Check sheet for the modelled part. Datum: model origin and axes. Units: mm. Face numbers are marked on the shaded views. A direction names the side the tool comes from. Coordinates: 2 decimals unless noted, no trailing zeros. Order: outer loops, then holes, each group sorted by start corner. A loop starts at its lowest first (then second) coordinate and runs counter-clockwise, first axis right, second up.
1. Draft check along X on the marked faces 3, 4, 5 and 6. Enter one of: released by +X, released by -X, zero draft, split by the parting line, or undercut.
2. Cross-section at A-A (y = 0). Enter the section's corners in (x, z), then the cut area to 3 significant figures.
3. Cross-section at B-B (x = -4.4). Enter the section's corners in (y, z), then the cut area to 3 significant figures.
4. Cross-section at C-C (y = -7.7). Enter the section's corners in (x, z), then the cut area to 3 significant figures.
5. Set-up check for the marked faces 1 and 2: record each of +Z, -Z, +X, -X, +Y, -Y from which the full face is reachable in a straight line by a thin tool's end or side.
6. Thickness scan on line 1 (Y direction, x = 0, z = 0.7); line 2 (X direction, y = 4.5, z = 5); line 3 (Y direction, x = -4.4, z = 0.9). Record the ranges inside material, lowest first.
7. Gauge pin test, flat ends, axial feed: pin 1 Ø1.6 at (x, y) = (-6.22, 0) entering from -Z; pin 2 Ø2.5 at (x, y) = (0, 6.22) entering from +Z; pin 3 Ø3 at (x, y) = (2.5, -1.5) entering from -Z. Record the tip position at first contact, or that the pin passes through.
8. Cross-section at D-D (z = 3.5). Enter the section's corners in (x, y).
Autodesk Inventor part; units mm, degrees
ref_plane "YZ Plane" through (0, 0, 0) normal (1, 0, 0) x (0, 1, 0)
ref_plane "XZ Plane" through (0, 0, 0) normal (0, 1, 0) x (-1, 0, 0)
ref_plane "XY Plane" through (0, 0, 0) normal (0, 0, 1) x (1, 0, 0)
sketch "スケッチ1" plane through (0, 0, 0) normal (0, 0, 1) x (1, 0, 0)
  line L0 (11, -10) -> (-11, -10)
  line L1 (-11, -10) -> (-11, 10)
  line L2 (-11, 10) -> (11, 10)
  line L3 (11, 10) -> (11, -10)
  line L4 (11, -10) -> (-11, 10) construction
  line L5 (-11, -10) -> (11, 10) construction
  point P0 (0, 0)
  dimension "d2" = 22
  dimension "d3" = 20
extrude "プレート1" add sketch "スケッチ1" along normal blind 1.2
sketch "スケッチ2" plane through (-11, -10, 1.2) normal (-1, 0, 0) x (0, -1, 0)
  line L0 (-20, 0) -> (0, 0)
  line L1 (0, 0) -> (0, 6.5)
  line L2 (0, 6.5) -> (-20, 6.5)
  line L3 (-20, 6.5) -> (-20, 0)
edge flange "フランジ1" height 7.7 angle 90 thickness 1.2 bend radius 0.5 thickness toward (-1, 0, 0) relief tear relief width 1.2 relief depth 0.6 corner gap 1.2 corner form 0 edges at (-11, 0, 1.2) (11, 0, 1.2) wall of the first edge with corners at (-11, 10, 1.2) (-11, -10, 1.2) (-11, -10, 7.7) (-11, 10, 7.7)
bend "曲げ1"
corner "コーナー1"
sketch "スケッチ3" plane through (0, 0, 1.2) normal (0, 0, 1) x (1, 0, 0)
  circle A0 centre (0, 0) radius 4.05
  dimension "d15" = 8.1
extrude "押し出し1" cut sketch "スケッチ3" against normal through all
sketch "スケッチ4" plane through (0, 0, 1.2) normal (0, 0, 1) x (1, 0, 0)
  line L0 (0, 0) -> (0, 6.2225)
  circle A0 centre (0, 6.2225) radius 0.9423
  circle A1 centre (-4.4, 4.4) radius 0.9423
  circle A2 centre (-6.2225, 0) radius 0.9423
  circle A3 centre (-4.4, -4.4) radius 0.9423
  circle A4 centre (0, -6.2225) radius 0.9423
  circle A5 centre (4.4, -4.4) radius 0.9423
  circle A6 centre (6.2225, 0) radius 0.9423
  circle A7 centre (4.4, 4.4) radius 0.9423
  dimension "d20" = 360
  dimension "d22" = 8.8
hole "穴1" at (0, 6.2225, 1.2) at (4.4, 4.4, 1.2) at (6.2225, 0, 1.2) at (4.4, -4.4, 1.2) at (0, -6.2225, 1.2) at (-4.4, -4.4, 1.2) at (-6.2225, 0, 1.2) at (-4.4, 4.4, 1.2) direction (0, 0, -1) diameter 2 end through all
sketch "スケッチ5" plane through (12.2, -10, 7.7) normal (1, 0, 0) x (0, 0, -1)
  line L0 (2.2, 2.3) -> (2.2, 17.7)
  line L1 (6.5, 9) -> (6.5, 11)
  line L2 (6.5, 2.7775) -> (6.5, 4.7775)
  line L3 (6.5, 9) -> (6.5, 11)
  line L4 (6.5, 15.2225) -> (6.5, 17.2225)
  line L5 (6.5, 13.4) -> (6.5, 15.4)
  line L6 (6.5, 4.6) -> (6.5, 6.6)
  line L7 (6.5, 4.6) -> (6.5, 6.6)
  line L8 (6.5, 13.4) -> (6.5, 15.4)
  line L9 (6.5, 5.95) -> (6.5, 14.05)
  line L10 (6.5, 0) -> (6.5, 20)
  line L11 (6.5, 20) -> (6.5, 0)
  line L12 (7.7, 10) -> (2.2, 10)
  dimension "d30" = 15.4
  dimension "d31" = 4.3
hole "穴2" at (12.2, 7.7, 5.5) at (12.2, -7.7, 5.5) direction (-1, 0, 0) diameter 1.321 end through all
sketch "スケッチ6" plane through (12.2, -10, 7.7) normal (1, 0, 0) x (0, 0, -1)
  circle A0 centre (2.2, 17.7) radius 0.6605
  circle A1 centre (2.2, 2.3) radius 0.6605
  line L0 (6, 0) -> (6, 20)
  line L1 (0, 20) -> (6, 20)
  line L2 (0, 0) -> (0, 20)
  line L3 (6, 0) -> (0, 0)
  point P0 (7.7, 10)
hole "穴3" at (12.2, -7.7, 5.5) at (12.2, 7.7, 5.5) direction (-1, 0, 0) diameter 1.7 depth 10 tip angle 118
sketch "スケッチ7" plane through (-12.2, -10, 7.7) normal (-1, 0, 0) x (0, 0, 1)
  circle A0 centre (-2.2, 17.7) radius 0.6605
  circle A1 centre (-2.2, 2.3) radius 0.6605
  line L0 (-6, 20) -> (-6, 0)
  line L1 (0, 0) -> (-6, 0)
  line L2 (0, 20) -> (0, 0)
  line L3 (-6, 20) -> (0, 20)
  line L4 (-6.5, 11) -> (-6.5, 9)
  line L5 (-6.5, 4.7775) -> (-6.5, 2.7775)
  line L6 (-6.5, 11) -> (-6.5, 9)
  line L7 (-6.5, 17.2225) -> (-6.5, 15.2225)
  line L8 (-6.5, 15.4) -> (-6.5, 13.4)
  line L9 (-6.5, 6.6) -> (-6.5, 4.6)
  line L10 (-6.5, 6.6) -> (-6.5, 4.6)
  line L11 (-6.5, 15.4) -> (-6.5, 13.4)
  line L12 (-6.5, 14.05) -> (-6.5, 5.95)
  line L13 (-6.5, 0) -> (-6.5, 20)
  line L14 (-6.5, 20) -> (-6.5, 0)
  line L15 (-6.5, 10) -> (4, 10)
  circle A2 centre (4, 10) radius 6.5
  point P0 (-7.7, 10)
  dimension "d46" = 10.5
  dimension "d47" = 13
extrude "押し出し2" cut sketch "スケッチ7" against normal up to surface (1.2 mm away) contours A2 L2 L15 | L15 L2 A2 | A2 L2
fillet "コーナーR1" radius 0.5 6 edges at (-11.6, -10, 7.7) (11.6, -10, 7.7) (11.6, 10, 7.7) (-11.6, 10, 7.7) (-11.6, -5.1235, 7.7) (-11.6, 5.1235, 7.7)
equation "\"d28\" = Thickness"
equation "\"d5\" = BendReliefWidth"
equation "\"d6\" = BendReliefDepth"
equation "\"d7\" = MinimumRemnant"
equation "\"d8\" = BendRadius"
equation "\"d12\" = CornerReliefSize"
equation "\"d13\" = GapSize"
equation "\"d14\" = JacobiRadiusSize"
equation "\"BendRadius\" = Thickness"
equation "\"BendReliefWidth\" = Thickness"
equation "\"BendReliefDepth\" = 0.5 * Thickness"
equation "\"CornerReliefSize\" = 4 * Thickness"
equation "\"MinimumRemnant\" = 2 * Thickness"
equation "\"TransitionRadius\" = BendRadius"
equation "\"JacobiRadiusSize\" = BendRadius"
equation "\"GapSize\" = Thickness"
equation "\"d4\" = BendRadius"
properties part number "G-ROBOTSアルミブラケットC" material "アルミニウム 6061"
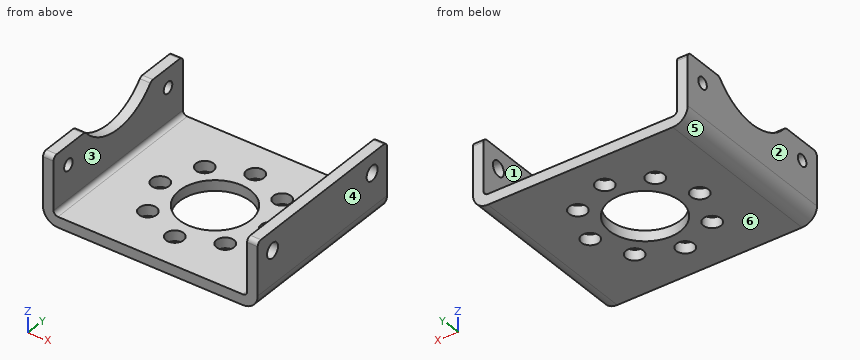
Data:
1. face 3: undercut
1. face 4: released by +X
1. face 5: released by -X
1. face 6: zero draft
2. outline: (-12.2, 1.7) arc R1.7 ccw to (-10.5, 0) - (-7.22, 0) - (-7.22, 1.2) - (-10.5, 1.2) arc R0.5 cw to (-11, 1.7) - (-11, 5.2) - (-12.2, 5.2) - close; (-5.22, 0) - (-4.05, 0) - (-4.05, 1.2) - (-5.22, 1.2) - close; (4.05, 0) - (5.22, 0) - (5.22, 1.2) - (4.05, 1.2) - close; (7.22, 0) - (10.5, 0) arc R1.7 ccw to (12.2, 1.7) - (12.2, 7.7) - (11, 7.7) - (11, 1.7) arc R0.5 cw to (10.5, 1.2) - (7.22, 1.2) - close
2. area: 26.2 mm2
3. outline: (-10, 0) - (-5.4, 0) - (-5.4, 1.2) - (-10, 1.2) - close; (-3.4, 0) - (3.4, 0) - (3.4, 1.2) - (-3.4, 1.2) - close; (5.4, 0) - (10, 0) - (10, 1.2) - (5.4, 1.2) - close
3. area: 19.2 mm2
4. outline: (-12.2, 1.7) arc R1.7 ccw to (-10.5, 0) - (10.5, 0) arc R1.7 ccw to (12.2, 1.7) - (12.2, 4.65) - (11, 4.65) - (11, 1.7) arc R0.5 cw to (10.5, 1.2) - (-10.5, 1.2) arc R0.5 cw to (-11, 1.7) - (-11, 4.84) - (-12.2, 4.84) - close; (-12.2, 6.16) - (-11, 6.16) - (-11, 7.7) - (-12.2, 7.7) - close; (11, 6.35) - (12.2, 6.35) - (12.2, 7.7) - (11, 7.7) - close
4. area: 40.1 mm2
5. face 1: +Z, +Y, -Y
5. face 2: +Z, -Z, -X, +Y, -Y
6. line 1: y = -10 to -7.22, -5.22 to -4.05, 4.05 to 5.22, 7.22 to 10
6. line 2: x = -12.2 to -11, 11 to 12.2
6. line 3: y = -10 to -5.4, -3.4 to 3.4, 5.4 to 10
7. pin 1: passes through
7. pin 2: stops at z = 1.2
7. pin 3: stops at z = 0
8. outline: (-12.2, -10) - (-11, -10) - (-11, 10) - (-12.2, 10) - close; (11, -10) - (12.2, -10) - (12.2, 10) - (11, 10) - close
